from build123d import *

# Parameters (mm, degrees)
F0_W     = 76.930061
F0_H     = 65.020956
F1_DEPTH = 20
F2_T     = -10
F4_D     = 5
F5_W     = 5.887607
F5_H     = 38.850113
F5_H_2   = 38.850112
F5_W_2   = 5.887608
F6_DEPTH = 10


with BuildPart() as f1:
    # F0 (on Front) → F1 (new body)
    with BuildSketch(Plane.XZ):
        with Locations((-0.03422, 1.129311)):
            Rectangle(F0_W, F0_H)
    extrude(amount=F1_DEPTH)

    # F2
    f2_openings = [f1.faces().sort_by_distance(p)[0] for p in [
        (-0.034221, -20, 1.129311),
    ]]
    offset(amount=F2_T, openings=f2_openings)

    # F4 (through all)
    with Locations(Plane.XZ.offset(10)):
        with Locations((-24.052991, 19.35718), (23.135278, -16.549327)):
            Hole(F4_D / 2)

    # F5 (on face) → F6 (join)
    with BuildSketch(Plane.XZ.offset(10)):
        with Locations((-17.145664, 4.214733)):
            Rectangle(F5_W, F5_H)
        with Locations((-8.301861, -1.956111)):
            Rectangle(F5_W, F5_H_2)
        with Locations((16.974628, -1.956111)):
            Rectangle(F5_W_2, F5_H_2)
        with Locations((6.936476, 4.405541)):
            Rectangle(F5_W, F5_H)
    extrude(amount=F6_DEPTH)


solid = f1.part
Verification items for the finished model (mm, model axes). A direction names the side the tool comes from. Coordinates: 2 decimals unless noted, no trailing zeros. Write each loop counter-clockwise with the first axis right and the second up, starting at its lowest first coordinate (ties: lowest second). Pieces come first, ordered by that corner, then holes. Notation, with made-up numbers: (-12.5, 48.25) -> (-8.5, 48.25) arc R18 ccw to (-8.5, 75.25) -> close; hole circle Ø6 at (-0.5, 42.25). An arc over 180 degrees is marked (long way). One line per item, written item: value. Start each with the question number.
Q1. Cross-section at A-A on y = -12. Enter the section's corners in (x, z), and give its area (3 significant figures).
Q2. Access from +Z, -Z, +X, -X, +Y, -Y to the whole of each face (thin tool, end or side, straight path). Record for faces 4 (the cylindrical face through (21.982, -4.93, -18.767)), 5 (the flat face through (-8, -15, 17.469)).
Q3. Cross-section at C-C on x = 3. Enter the section's corners in (y, z).
Q4. Go/stop test with a flat-tipped pin: P1, Ø1, axis at x = -23.5, z = 14.5, coming from the -Y side. Record where the tip stops, or that it passes through.
Q5. Mould release check, pull along X, two halves, no side actions. Record for faces 1 (the flat face through (17, -15, 17.469)), 2 (the flat face through (-1, -10, 33.64)), 3 (the flat face through (-5, -15, 23.64)): pulls with the +X half, pulls with the -X half, needs draft (parallel to the pull), parting line crosses it, or undercut.
Q6. Cross-section at D-D on z = 1. Enter the section's corners in (x, y), and give its area (3 significant figures).
Q7. Thickness scan on L1, parallel to X at y = -10.75, z = 3.5; L2, parallel to X at y = -14.5, z = -16.5; L3, parallel to Z at x = 24, y = -10.25. Record the ranges inside material, lowest first. Write a range as from..to.
Q8. Cross-section at B-B on z = 21. Enter the section's corners in (x, y), and give its area (3 significant figures).
Checked values:
1. outline: (-38.5, -31.38) -> (38.43, -31.38) -> (38.43, 33.64) -> (-38.5, 33.64) -> close; hole (-28.5, -21.38) -> (-11.25, -21.38) -> (-11.25, 17.47) -> (-5.36, 17.47) -> (-5.36, -21.38) -> (14.03, -21.38) -> (14.03, 17.47) -> (19.92, 17.47) -> (19.92, -21.38) -> (28.43, -21.38) -> (28.43, 23.64) -> (9.88, 23.64) -> (9.88, -15.02) -> (3.99, -15.02) -> (3.99, 23.64) -> (-14.2, 23.64) -> (-14.2, -15.21) -> (-20.09, -15.21) -> (-20.09, 23.64) -> (-28.5, 23.64) -> close
1. area: 3,350 mm²
2. face 4: +Y, -Y
2. face 5: -Y
3. outline: (-20, -31.38) -> (0, -31.38) -> (0, 33.64) -> (-20, 33.64) -> (-20, 23.64) -> (-10, 23.64) -> (-10, -21.38) -> (-20, -21.38) -> close
4. P1: stops at y = -10
5. face 1: undercut
5. face 2: needs draft
5. face 3: undercut
6. outline: (-38.5, -20) -> (-28.5, -20) -> (-28.5, -10) -> (-20.09, -10) -> (-20.09, -20) -> (-14.2, -20) -> (-14.2, -10) -> (-11.25, -10) -> (-11.25, -20) -> (-5.36, -20) -> (-5.36, -10) -> (3.99, -10) -> (3.99, -20) -> (9.88, -20) -> (9.88, -10) -> (14.03, -10) -> (14.03, -20) -> (19.92, -20) -> (19.92, -10) -> (28.43, -10) -> (28.43, -20) -> (38.43, -20) -> (38.43, 0) -> (-38.5, 0) -> close
6. area: 1,200 mm²
7. L1: x = -38.5..-28.5, -20.09..-14.2, -11.25..-5.36, 3.99..9.88, 14.03..19.92, 28.43..38.43
7. L2: x = -38.5..-28.5, -11.25..-5.36, 14.03..19.92, 28.43..38.43
7. L3: z = -31.38..-21.38, 23.64..33.64
8. outline: (-38.5, -20) -> (-28.5, -20) -> (-28.5, -10) -> (-25.94, -10) -> (-25.94, 0) -> (-38.5, 0) -> close; (-22.17, -10) -> (-20.09, -10) -> (-20.09, -20) -> (-14.2, -20) -> (-14.2, -10) -> (3.99, -10) -> (3.99, -20) -> (9.88, -20) -> (9.88, -10) -> (28.43, -10) -> (28.43, -20) -> (38.43, -20) -> (38.43, 0) -> (-22.17, 0) -> close
8. area: 1,050 mm²
